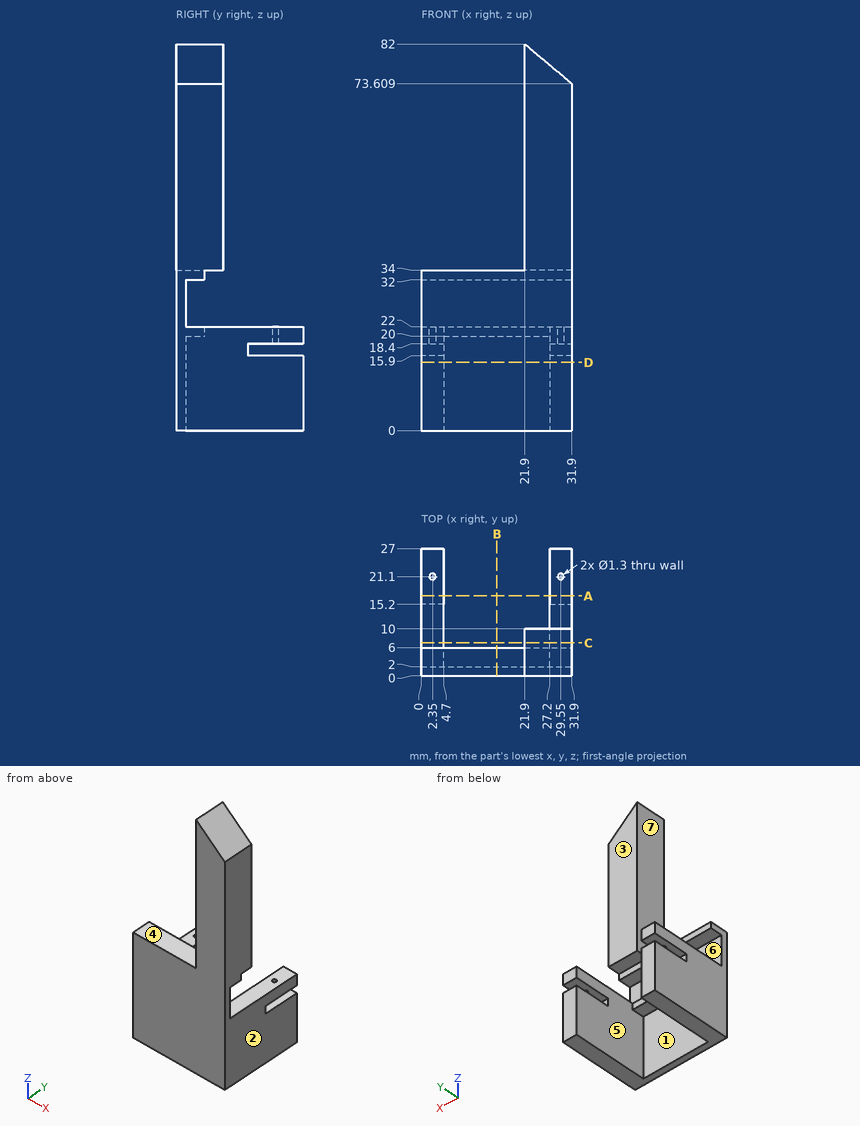
Source: three-view drawing plus pictorial views. Frame: mm from the lowest corner of the part. A direction names the side the tool comes from. Round coordinates to 2 decimals unless told otherwise and drop trailing zeros. Loops run counter-clockwise (first coordinate to the right, second up) from the corner with the lowest first, then second, coordinate; pieces in that order, holes last.
1. Access query for the marked faces 1, 2, 3 and 4. Directions: +Z, -Z, +X, -X, +Y, -Y. A direction counts if a zero-diameter tool reaches every point of the face in a straight line with its end or side. Return the directions, or none.
2. Section query D-D on z = 14.5. Output: boundary loops of the cut face in (x, y).
3. Section query C-C on y = 7. Output: boundary loops of the cut face in (x, z), and give its area (3 significant figures).
4. Section query B-B on x = 16. Output: boundary loops of the cut face in (y, z).
5. Mould query, pull axis X, two halves, no side actions, for the marked faces 5, 6 and 7. Classes: released by +X, released by -X, zero draft, split by the parting line, or undercut.
6. Contact query for flat-ended pins moving along their axis: pin 1 (4 mm diameter, centred on y = 8, z = 39.5, fed in from -X); pin 2 (5 mm diameter, centred on x = 11.5, y = 2, fed in from +Z); pin 3 (3 mm diameter, centred on x = 24.5, z = 67.5, fed in from +Y). Output: stop coordinate, or through.
7. Ray query, L1, parallel to Z at x = 12.5, y = 4.75; L2, parallel to Z at x = 29.5, y = 24; L3, parallel to Y at x = 29.55, z = 20.6. Return the intervals inside material, ascending.
8. Section query A-A on y = 17. Output: boundary loops of the cut face in (x, z).
Answers below:
1. face 1: -Z, +Y
1. face 2: +Z, -Z, +X, +Y, -Y
1. face 3: +Z, +X, -X, +Y
1. face 4: +Z, -X, +Y, -Y
2. outline: (0, 0) - (31.9, 0) - (31.9, 27) - (27.2, 27) - (27.2, 2) - (4.7, 2) - (4.7, 27) - (0, 27) - close
3. outline: (0, 0) - (4.7, 0) - (4.7, 22) - (0, 22) - close; (21.9, 34) - (31.9, 34) - (31.9, 73.61) - (21.9, 82) - close; (27.2, 0) - (31.9, 0) - (31.9, 22) - (27.2, 22) - close
3. area: 645 mm2
4. outline: (0, 0) - (2, 0) - (2, 20) - (6, 20) - (6, 22) - (2, 22) - (2, 32) - (6, 32) - (6, 34) - (0, 34) - close
5. face 5: undercut
5. face 6: zero draft
5. face 7: released by -X
6. pin 1: stops at x = 21.9
6. pin 2: stops at z = 34
6. pin 3: stops at y = 10
7. L1: z = 20 to 22, 32 to 34
7. L2: z = 0 to 15.9, 18.4 to 22
7. L3: y = 0 to 20.45, 21.75 to 27
8. outline: (0, 0) - (4.7, 0) - (4.7, 15.9) - (0, 15.9) - close; (0, 18.4) - (4.7, 18.4) - (4.7, 22) - (0, 22) - close; (27.2, 0) - (31.9, 0) - (31.9, 15.9) - (27.2, 15.9) - close; (27.2, 18.4) - (31.9, 18.4) - (31.9, 22) - (27.2, 22) - close
